Check sheet for the modelled part. Datum: model origin and axes. Units: mm. Face numbers are marked on the shaded views. A direction names the side the tool comes from. Round coordinates to 2 decimals unless told otherwise and drop trailing zeros. Write each loop counter-clockwise with the first axis right and the second up, starting at its lowest first coordinate (ties: lowest second). Pieces come first, ordered by that corner, then holes.
Item 1: Section check B-B, the plane z = 15.5. Record the cut outline in (x, y) (3 decimals).
Item 2: Section check C-C, the plane x = 7. Record the cut outline in (y, z) (3 decimals).
Item 3: Section check D-D, the plane y = 13.5. State how many separate pieces and enclosed holes the cut face has, plus the area to 3 significant figures.
Item 4: Section check A-A, the plane y = 19.05. Record the cut outline in (x, z) (3 decimals), plus the area to 3 significant figures.
Item 5: Set-up check for the marked faces 1, 2 and 3: record each of +Z, -Z, +X, -X, +Y, -Y from which the full face is reachable in a straight line by a thin tool's end or side.
Item 6: Material ranges on line 1 along Y through (x, z) = (2.5, 7.5); line 2 along Z through (x, y) = (8, 22.75) (3 decimals), recorded low to high.
Item 7: Depth check by flat-ended pin: pin 1 (4 mm diameter, centred on y = 21.336, z = 7.239, fed in from +X) (3 decimals); pin 2 (8 mm diameter, centred on y = 21.5, z = 5.5, fed in from +X); pin 3 (2 mm diameter, centred on x = 12.5, y = 6.5, fed in from +Z) (3 decimals). Enter the tip coordinate at first touch or a pass-through.
from build123d import *

# Parameters (mm, degrees)
BOSS_EXTRUDE1_DEPTH   = 25.4
F_6_CLEARANCE_HOLE1_D = 3.6576
CHAMFER1_SIZE         = 2.54
F_4_40_TAPPED_HOLE1_D = 2.2606
SKETCH8_W             = 7.62
SKETCH8_H             = 12.7
BOSS_EXTRUDE2_DEPTH   = 3.175


with BuildPart() as part:
    # Sketch1 → Boss-Extrude1 (new body)
    with BuildSketch(Plane(origin=(0, 0, 0), x_dir=(1, 0, 0), z_dir=(0, 1, 0))):
        Polygon((0, 0), (12.7, 0), (12.7, -3.175), (3.175, -3.175), (3.175, -19.05), (0, -19.05), align=None)
    extrude(amount=BOSS_EXTRUDE1_DEPTH)

    # #6 Clearance Hole1 (through all)
    with Locations(Plane.ZY):
        with Locations((7.239, 4.064), (7.239, 21.336), (14.986, 12.7)):
            Hole(F_6_CLEARANCE_HOLE1_D / 2)

    # Chamfer1
    chamfer1_edges = [part.edges().sort_by_distance(p)[0] for p in [
        (12.7, 25.4, 1.5875),
        (12.7, 0, 1.5875),
        (1.5875, 25.4, 19.05),
        (1.5875, 0, 19.05),
    ]]
    chamfer(chamfer1_edges, length=CHAMFER1_SIZE)

    # #4-40 Tapped Hole1 (through all)
    with Locations(Plane(origin=(0, 0, 0), x_dir=(-1, 0, 0), z_dir=(0, 0, -1))):
        with Locations((-6.8499944, 6.35), (-6.8499944, 12.7), (-6.8499944, 19.05)):
            Hole(F_4_40_TAPPED_HOLE1_D / 2)

    # Sketch8 → Boss-Extrude2 (add)
    with BuildSketch(Plane(origin=(0, 0, 0), x_dir=(-1, 0, 0), z_dir=(0, 0, -1))):
        with Locations((-13.97, 6.35)):
            Rectangle(SKETCH8_W, SKETCH8_H)
    extrude(amount=-BOSS_EXTRUDE2_DEPTH)


solid = part.part
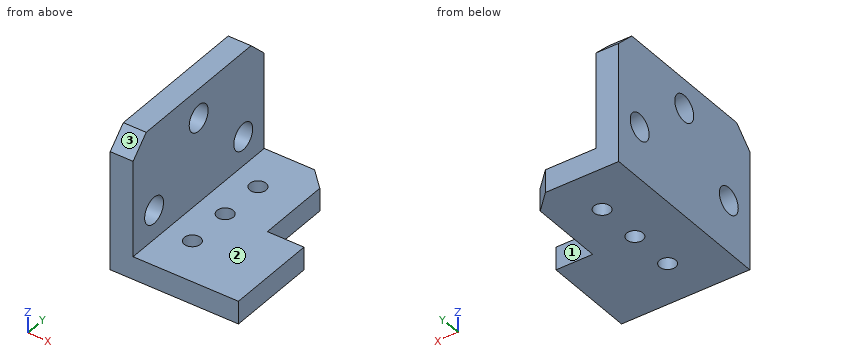
Values found:
1. outline: (0, 0) - (3.175, 0) - (3.175, 10.945) - (0, 10.945) - close; (0, 14.455) - (3.175, 14.455) - (3.175, 25.4) - (0, 25.4) - close
2. outline: (0, 0) - (5.23, 0) - (5.23, 3.175) - (0, 3.175) - close; (7.47, 0) - (11.58, 0) - (11.58, 3.175) - (7.47, 3.175) - close; (13.82, 0) - (17.93, 0) - (17.93, 3.175) - (13.82, 3.175) - close; (20.17, 0) - (25.4, 0) - (25.4, 3.175) - (20.17, 3.175) - close
3. separate pieces: 3
3. enclosed holes: 0
3. area: 75.2 mm2
4. outline: (0, 0) - (5.72, 0) - (5.72, 3.175) - (3.175, 3.175) - (3.175, 19.05) - (0, 19.05) - close; (7.98, 0) - (12.7, 0) - (12.7, 3.175) - (7.98, 3.175) - close
4. area: 83.5 mm2
5. face 1: +Z, -Z, +X, +Y
5. face 2: +Z, +X, +Y, -Y
5. face 3: +Z, +X, -X, -Y
6. line 1: y = 0 to 2.25, 5.87 to 19.53, 23.15 to 25.4
6. line 2: z = 0 to 3.175
7. pin 1: stops at x = 3.175
7. pin 2: stops at x = 12.7
7. pin 3: stops at z = 3.175
